Design review of the part built by this model. Coordinates are the model's own, in mm. A direction names the side the tool comes from. Give positions to 0.01 mm unless a question says otherwise; leave off trailing zeros. Write each loop counter-clockwise with the first axis right and the second up, starting at its lowest first coordinate (ties: lowest second). Pieces come first, ordered by that corner, then holes.
```python
from build123d import *

# Parameters (mm, degrees)
SKETCH_1_W          = 48
SKETCH_1_H          = 38
EXTRUDE_1_DEPTH     = 1.6
SKETCH_5_R          = 1
SKETCH_5_R_2        = 0.475
CUT_EXTRUDE_1_DEPTH = 1.6
SKETCH_8_W          = 1.6
SKETCH_8_H          = 19
EXTRUDE_3_DEPTH     = 4
SKETCH_9_W          = 6
SKETCH_9_H          = 1.6
EXTRUDE_4_DEPTH     = 3
CUT_EXTRUDE_2_REACH = 37.254
SKETCH_10_R         = 0.45


with BuildPart() as part:
    # 草图1 → 凸台-拉伸1 (new body)
    with BuildSketch(Plane.XY):
        with Locations((3.5, 0)):
            Rectangle(SKETCH_1_W, SKETCH_1_H)
    extrude(amount=-EXTRUDE_1_DEPTH)

    # 草图5 → 切除-拉伸1 (cut)
    with BuildSketch(Plane.XY):
        with Locations((-9.14, 15.85)):
            Circle(SKETCH_5_R)
        with Locations((11.06, 15.85)):
            Circle(SKETCH_5_R)
        with Locations((22.6, 10.35)):
            Circle(SKETCH_5_R)
        with Locations((22.6, -10.35)):
            Circle(SKETCH_5_R)
        with Locations((-11.89, 8.89)):
            Circle(SKETCH_5_R_2)
        with Locations((-9.35, 8.89)):
            Circle(SKETCH_5_R_2)
        with Locations((-6.81, 8.89)):
            Circle(SKETCH_5_R_2)
        with Locations((-4.27, 8.89)):
            Circle(SKETCH_5_R_2)
        with Locations((-11.89, 11.43)):
            Circle(SKETCH_5_R_2)
        with Locations((-9.35, 11.43)):
            Circle(SKETCH_5_R_2)
        with Locations((-6.81, 11.43)):
            Circle(SKETCH_5_R_2)
        with Locations((-4.27, 11.43)):
            Circle(SKETCH_5_R_2)
        with Locations((-1.73, 11.43)):
            Circle(SKETCH_5_R_2)
        with Locations((0.81, 11.43)):
            Circle(SKETCH_5_R_2)
        with Locations((3.35, 11.43)):
            Circle(SKETCH_5_R_2)
        with Locations((-1.73, 8.89)):
            Circle(SKETCH_5_R_2)
        with Locations((0.81, 8.89)):
            Circle(SKETCH_5_R_2)
        with Locations((3.35, 8.89)):
            Circle(SKETCH_5_R_2)
        with Locations((5.89, 8.89)):
            Circle(SKETCH_5_R_2)
        with Locations((8.43, 8.89)):
            Circle(SKETCH_5_R_2)
        with Locations((5.89, 11.43)):
            Circle(SKETCH_5_R_2)
        with Locations((8.43, 11.43)):
            Circle(SKETCH_5_R_2)
        with Locations((10.8, 11.43)):
            Circle(SKETCH_5_R_2)
        with Locations((10.8, 8.89)):
            Circle(SKETCH_5_R_2)
        with Locations((10.8, 6.35)):
            Circle(SKETCH_5_R_2)
        with Locations((10.8, 3.81)):
            Circle(SKETCH_5_R_2)
        with Locations((10.8, 1.27)):
            Circle(SKETCH_5_R_2)
        with Locations((10.8, -1.27)):
            Circle(SKETCH_5_R_2)
        with Locations((10.8, -3.81)):
            Circle(SKETCH_5_R_2)
        with Locations((10.8, -6.35)):
            Circle(SKETCH_5_R_2)
        with Locations((-11.89, -8.89)):
            Circle(SKETCH_5_R_2)
        with Locations((-9.35, -8.89)):
            Circle(SKETCH_5_R_2)
        with Locations((-6.81, -8.89)):
            Circle(SKETCH_5_R_2)
        with Locations((-4.27, -8.89)):
            Circle(SKETCH_5_R_2)
        with Locations((-1.73, -8.89)):
            Circle(SKETCH_5_R_2)
        with Locations((0.81, -8.89)):
            Circle(SKETCH_5_R_2)
        with Locations((3.35, -8.89)):
            Circle(SKETCH_5_R_2)
        with Locations((5.89, -8.89)):
            Circle(SKETCH_5_R_2)
        with Locations((8.43, -8.89)):
            Circle(SKETCH_5_R_2)
        with Locations((10.8, -8.89)):
            Circle(SKETCH_5_R_2)
        with Locations((-11.89, -11.43)):
            Circle(SKETCH_5_R_2)
        with Locations((-9.35, -11.43)):
            Circle(SKETCH_5_R_2)
        with Locations((-6.81, -11.43)):
            Circle(SKETCH_5_R_2)
        with Locations((-4.27, -11.43)):
            Circle(SKETCH_5_R_2)
        with Locations((-1.73, -11.43)):
            Circle(SKETCH_5_R_2)
        with Locations((0.81, -11.43)):
            Circle(SKETCH_5_R_2)
        with Locations((3.35, -11.43)):
            Circle(SKETCH_5_R_2)
        with Locations((5.89, -11.43)):
            Circle(SKETCH_5_R_2)
        with Locations((8.43, -11.43)):
            Circle(SKETCH_5_R_2)
        with Locations((10.8, -11.43)):
            Circle(SKETCH_5_R_2)
        with Locations((3.5, 17.73)):
            Circle(SKETCH_5_R_2)
        with Locations((6.04, 17.73)):
            Circle(SKETCH_5_R_2)
        with Locations((0.96, 17.73)):
            Circle(SKETCH_5_R_2)
        with Locations((-4.12, 17.73)):
            Circle(SKETCH_5_R_2)
        with Locations((-1.58, 17.73)):
            Circle(SKETCH_5_R_2)
        with Locations((11.06, -15.85)):
            Circle(SKETCH_5_R)
        with Locations((-9.14, -15.85)):
            Circle(SKETCH_5_R)
    extrude(amount=-CUT_EXTRUDE_1_DEPTH, mode=Mode.SUBTRACT)

    # 草图8 → 凸台-拉伸3 (add)
    with BuildSketch(Plane.ZY.offset(20.5)):
        with Locations((-0.8, 0)):
            Rectangle(SKETCH_8_W, SKETCH_8_H)
    extrude(amount=EXTRUDE_3_DEPTH)

    # 草图9 → 凸台-拉伸4 (add)
    with BuildSketch(Plane.XZ.offset(19)):
        with Locations((-17.5, -0.8)):
            Rectangle(SKETCH_9_W, SKETCH_9_H)
        with Locations((24.5, -0.8)):
            Rectangle(SKETCH_9_W, SKETCH_9_H)
    extrude(amount=EXTRUDE_4_DEPTH)

    # 草图10 → 切除-拉伸2 (cut, up to next)
    with BuildSketch(Plane.XY, mode=Mode.PRIVATE) as cut_extrude_2_sk1:
        with Locations((-19, -19)):
            Circle(SKETCH_10_R)
    cut_extrude_2_tool1 = extrude(cut_extrude_2_sk1.sketch, amount=-CUT_EXTRUDE_2_REACH, mode=Mode.PRIVATE) & part.part
    # 草图10 → 切除-拉伸2 (cut, up to next)
    with BuildSketch(Plane.XY, mode=Mode.PRIVATE) as cut_extrude_2_sk2:
        with Locations((-16, -19)):
            Circle(SKETCH_10_R)
    cut_extrude_2_tool2 = extrude(cut_extrude_2_sk2.sketch, amount=-CUT_EXTRUDE_2_REACH, mode=Mode.PRIVATE) & part.part
    # 草图10 → 切除-拉伸2 (cut, up to next)
    with BuildSketch(Plane.XY, mode=Mode.PRIVATE) as cut_extrude_2_sk3:
        with Locations((-17.5, -21)):
            Circle(SKETCH_10_R)
    cut_extrude_2_tool3 = extrude(cut_extrude_2_sk3.sketch, amount=-CUT_EXTRUDE_2_REACH, mode=Mode.PRIVATE) & part.part
    # 草图10 → 切除-拉伸2 (cut, up to next)
    with BuildSketch(Plane.XY, mode=Mode.PRIVATE) as cut_extrude_2_sk4:
        with Locations((23, -19)):
            Circle(SKETCH_10_R)
    cut_extrude_2_tool4 = extrude(cut_extrude_2_sk4.sketch, amount=-CUT_EXTRUDE_2_REACH, mode=Mode.PRIVATE) & part.part
    # 草图10 → 切除-拉伸2 (cut, up to next)
    with BuildSketch(Plane.XY, mode=Mode.PRIVATE) as cut_extrude_2_sk5:
        with Locations((26, -19)):
            Circle(SKETCH_10_R)
    cut_extrude_2_tool5 = extrude(cut_extrude_2_sk5.sketch, amount=-CUT_EXTRUDE_2_REACH, mode=Mode.PRIVATE) & part.part
    # 草图10 → 切除-拉伸2 (cut, up to next)
    with BuildSketch(Plane.XY, mode=Mode.PRIVATE) as cut_extrude_2_sk6:
        with Locations((24.5, -21)):
            Circle(SKETCH_10_R)
    cut_extrude_2_tool6 = extrude(cut_extrude_2_sk6.sketch, amount=-CUT_EXTRUDE_2_REACH, mode=Mode.PRIVATE) & part.part
    add(cut_extrude_2_tool1.solids().sort_by_distance((-19, -19, 0))[0], mode=Mode.SUBTRACT)
    add(cut_extrude_2_tool2.solids().sort_by_distance((-16, -19, 0))[0], mode=Mode.SUBTRACT)
    add(cut_extrude_2_tool3.solids().sort_by_distance((-17.5, -21, 0))[0], mode=Mode.SUBTRACT)
    add(cut_extrude_2_tool4.solids().sort_by_distance((23, -19, 0))[0], mode=Mode.SUBTRACT)
    add(cut_extrude_2_tool5.solids().sort_by_distance((26, -19, 0))[0], mode=Mode.SUBTRACT)
    add(cut_extrude_2_tool6.solids().sort_by_distance((24.5, -21, 0))[0], mode=Mode.SUBTRACT)


solid = part.part
```
(1) Consider section C-C, the plane z = -0.55. Give the number of separate pieces and of enclosed holes in the cut face, then the cut area to 3 significant figures.
Resolved:
separate pieces: 1
enclosed holes: 63
area: 1,880 mm2
(2) Consider section A-A, the plane y = 10.35. Give the boundary of the cut face in (x, z), then the cut area to 3 significant figures.
Resolved:
outline: (-20.5, -1.6) - (21.6, -1.6) - (21.6, 0) - (-20.5, 0) - close; (23.6, -1.6) - (27.5, -1.6) - (27.5, 0) - (23.6, 0) - close
area: 73.6 mm2
(3) Consider section B-B, the plane y = -15.85. Give the boundary of the cut face in (x, z), then the cut area to 3 significant figures.
Resolved:
outline: (-20.5, -1.6) - (-10.14, -1.6) - (-10.14, 0) - (-20.5, 0) - close; (-8.14, -1.6) - (10.06, -1.6) - (10.06, 0) - (-8.14, 0) - close; (12.06, -1.6) - (27.5, -1.6) - (27.5, 0) - (12.06, 0) - close
area: 70.4 mm2
(4) Consider section D-D, the plane x = 17.5. Give the boundary of the cut face in (y, z).
Resolved:
outline: (-19, -1.6) - (19, -1.6) - (19, 0) - (-19, 0) - close
(5) Mouldability with a two-part tool opening along Y and no side actions: class faces 4 (the face through (-22, 9.5, -1)), 5 (the face through (11.6, 16.69, -0.79)), 6 (the face through (21.6, -10.3, -0.8)), 7 (the face through (1, -1, -1.6)) as pulls with the +Y half, pulls with the -Y half, needs draft (parallel to the pull), parting line crosses it, or undercut.
Resolved:
face 4: pulls with the +Y half
face 5: undercut
face 6: undercut
face 7: needs draft
(6) To check wall thickness, follow L1, parallel to Y at x = -12, z = -0.1; L2, parallel to X at y = 17.73, z = -0.35 (3 decimals); L3, parallel to Y at x = 22.5, z = -0.15. State the ranges of each line that lie inside material, in increasing order.
Resolved:
L1: y = -19 to -11.89, -10.97 to -9.35, -8.43 to 8.43, 9.35 to 10.97, 11.89 to 19
L2: x = -20.5 to -4.595, -3.645 to -2.055, -1.105 to 0.485, 1.435 to 3.025, 3.975 to 5.565, 6.515 to 27.5
L3: y = -22 to -11.34, -9.36 to 9.36, 11.34 to 19
(7) Clearance check with flat-ended pins moving along their axes: P1, Ø0.5, axis at y = -18, z = -1, coming from the -X side; P2, Ø0.8, axis at x = -1.5, z = -0.5, coming from the -Y side. State where each tip first meets the part, or that it passes through.
Resolved:
P1: stops at x = -20.5
P2: stops at y = -19
(8) Tool access review of faces 1 (the face through (-20.5, 14, -1)), 2 (the face through (-20.5, -16, -1)), 3 (the face through (-14.5, -20, -1)): name each direction out of +Z, -Z, +X, -X, +Y, -Y from which nothing blocks a thin tool from reaching the whole face with its end or side.
Resolved:
face 1: +Z, -Z, -X, +Y
face 2: +Z, -Z, -X, -Y
face 3: +Z, -Z, -Y
